from build123d import *

# Parameters (mm, degrees)
SKETCH1_W           = 58
SKETCH1_H           = 135
SKETCH1_R           = 16.5
SKETCH1_R_2         = 2.375
SKETCH1_R_3         = 2.65
BOSS_EXTRUDE1_DEPTH = 4


with BuildPart() as part:
    # Sketch1 → Boss-Extrude1 (new body)
    with BuildSketch(Plane(origin=(0, 0, 0), x_dir=(0, 0, -1), z_dir=(1, 0, 0))):
        Rectangle(SKETCH1_W, SKETCH1_H)
        with Locations((0, -6.5)):
            Circle(SKETCH1_R, mode=Mode.SUBTRACT)
        with Locations((23.57, 17.07)):
            Circle(SKETCH1_R_2, mode=Mode.SUBTRACT)
        with Locations((-23.57, 17.07)):
            Circle(SKETCH1_R_2, mode=Mode.SUBTRACT)
        with Locations((-23.57, -30.07)):
            Circle(SKETCH1_R_2, mode=Mode.SUBTRACT)
        with Locations((23.57, -30.07)):
            Circle(SKETCH1_R_2, mode=Mode.SUBTRACT)
        with Locations((-19, 57.5)):
            Circle(SKETCH1_R_3, mode=Mode.SUBTRACT)
        with Locations((19, 57.5)):
            Circle(SKETCH1_R_3, mode=Mode.SUBTRACT)
        with Locations((-19, -57.5)):
            Circle(SKETCH1_R_3, mode=Mode.SUBTRACT)
        with Locations((19, -57.5)):
            Circle(SKETCH1_R_3, mode=Mode.SUBTRACT)
    extrude(amount=BOSS_EXTRUDE1_DEPTH)


solid = part.part
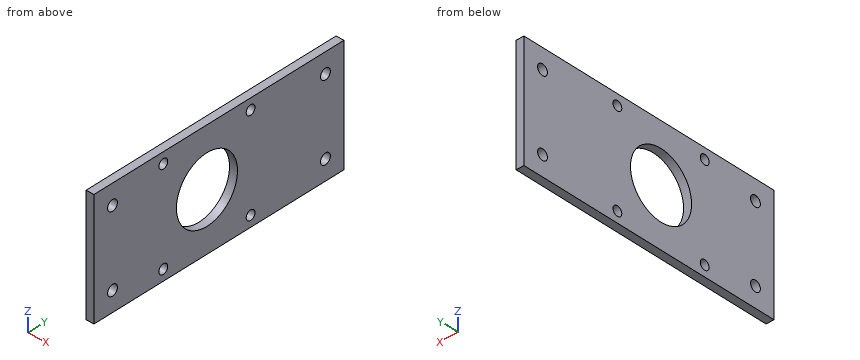
The model under review builds one solid part; all positions refer to its coordinate system, in mm. Round coordinates to 2 decimals unless told otherwise and drop trailing zeros. Order: outer loops, then holes, each group sorted by start corner. A loop starts at its lowest first (then second) coordinate and runs counter-clockwise, first axis right, second up. Notation, with made-up numbers: (49.5, -19.5) - (106.5, -19.5) arc R26 cw to (106.5, 14.5) - close; hole circle Ø11 at (-8, 3). An arc over 180 degrees is marked (long way). Use one line per item in the form item = value.
Q1. To check wall thickness, follow line 1 (Y direction, x = 1.3, z = 19); line 2 (Y direction, x = 2.75, z = 0); line 3 (Y direction, x = 1.35, z = -23.57) (3 decimals). State the ranges of each line that lie inside material, in increasing order.
Response values:
line_1 = -67.5 to -60.15, -54.85 to 54.85, 60.15 to 67.5
line_2 = -67.5 to -23, 10 to 67.5
line_3 = -67.5 to -32.445, -27.695 to 14.695, 19.445 to 67.5
Q2. Add section D-D on y = -6.5. Give the boundary of the cut face in (x, z), then the cut area to 3 significant figures.
Response values:
outline = (0, -29) - (4, -29) - (4, -16.5) - (0, -16.5) - close; (0, 16.5) - (4, 16.5) - (4, 29) - (0, 29) - close
area = 100 mm^2
Q3. Add section B-B on y = -30.07. Give the boundary of the cut face in (x, z) (3 decimals).
Response values:
outline = (0, -29) - (4, -29) - (4, -25.945) - (0, -25.945) - close; (0, -21.195) - (4, -21.195) - (4, 21.195) - (0, 21.195) - close; (0, 25.945) - (4, 25.945) - (4, 29) - (0, 29) - close
Q4. Add section A-A on z = 0. Give the boundary of the cut face in (x, y), then the cut area to 3 significant figures.
Response values:
outline = (0, -67.5) - (4, -67.5) - (4, -23) - (0, -23) - close; (0, 10) - (4, 10) - (4, 67.5) - (0, 67.5) - close
area = 408 mm^2
Q5. Add section C-C on z = 23.57. Give the boundary of the cut face in (x, y) (3 decimals), then the cut area to 3 significant figures.
Response values:
outline = (0, -67.5) - (4, -67.5) - (4, -32.445) - (0, -32.445) - close; (0, -27.695) - (4, -27.695) - (4, 14.695) - (0, 14.695) - close; (0, 19.445) - (4, 19.445) - (4, 67.5) - (0, 67.5) - close
area = 502 mm^2
